```python
from build123d import *

# Parameters (mm, degrees)
BOSS_EXTRUDE1_DEPTH = 8


with BuildPart() as part:
    # Sketch1 → Boss-Extrude1 (new body)
    with BuildSketch(Plane.XY):
        with BuildLine():
            Line((1, 0), (19, 0))
            ThreePointArc((19, 0), (19.707106781, 0.292893219), (20, 1))
            Line((20, 1), (20, 56.5))
            ThreePointArc((20, 56.5), (19.707106781, 57.207106781), (19, 57.5))
            Line((19, 57.5), (1, 57.5))
            ThreePointArc((1, 57.5), (0.292893219, 57.207106781), (0, 56.5))
            Line((0, 56.5), (0, 50.5))
            ThreePointArc((0, 50.5), (0.292893219, 49.792893219), (1, 49.5))
            Line((1, 49.5), (10, 49.5))
            Line((10, 49.5), (10, 41.5))
            Line((10, 41.5), (1, 41.5))
            ThreePointArc((1, 41.5), (0.292893219, 41.207106781), (0, 40.5))
            Line((0, 40.5), (0, 19))
            ThreePointArc((0, 19), (0.292893219, 18.292893219), (1, 18))
            Line((1, 18), (10, 18))
            Line((10, 18), (10, 10))
            Line((10, 10), (1, 10))
            ThreePointArc((1, 10), (0.292893219, 9.707106781), (0, 9))
            Line((0, 9), (0, 1))
            ThreePointArc((0, 1), (0.292893219, 0.292893219), (1, 0))
        make_face()
    extrude(amount=BOSS_EXTRUDE1_DEPTH)


solid = part.part
```
Input: part model. Units: mm. Frame: model coordinates. A direction names the side the tool comes from. Coordinates: 2 decimals unless noted, no trailing zeros. Write each loop counter-clockwise with the first axis right and the second up, starting at its lowest first coordinate (ties: lowest second). Pieces come first, ordered by that corner, then holes. Notation, with made-up numbers: (3.5, 66) -> (22.5, 66) arc R15 cw to (22.5, 85) -> close; hole circle Ø8 at (64, 75.25). An arc over 180 degrees is marked (long way). Answer as a JSON object with one key per item and string values.
1. First-contact query: P1, Ø4, axis at y = 44, z = 6, coming from the -X side. Flat tip, straight axial feed; report the tip coordinate or a pass-through.
Result set:
{"P1": "stops at x = 10"}
2. Access query for faces 1 (the face through (0.301, 41.215, 3.944)), 2 (the face through (0, 30, 4)). Directions: +Z, -Z, +X, -X, +Y, -Y. A direction counts if a zero-diameter tool reaches every point of the face in a straight line with its end or side. Return the directions, or none.
Result set:
{"face 1": "+Z, -Z, -X", "face 2": "+Z, -Z, -X, +Y, -Y"}
3. Section A-A on x = 2.5. Return the cut outline in (y, z).
Result set:
{"outline": "(0, 0) -> (10, 0) -> (10, 8) -> (0, 8) -> close; (18, 0) -> (41.5, 0) -> (41.5, 8) -> (18, 8) -> close; (49.5, 0) -> (57.5, 0) -> (57.5, 8) -> (49.5, 8) -> close"}
4. Section C-C on y = 13.5. Return the cut outline in (x, z).
Result set:
{"outline": "(10, 0) -> (20, 0) -> (20, 8) -> (10, 8) -> close"}
5. Material intervals for line 1 (Y direction, x = 6.75, z = 2.5); line 2 (X direction, y = 45, z = 3.75); line 3 (X direction, y = 18.5, z = 6.5), sorted ascending. Write a range as from..to.
Result set:
{"line 1": "y = 0..10, 18..41.5, 49.5..57.5", "line 2": "x = 10..20", "line 3": "x = 0.13..20"}
6. Section B-B on z = 6. Return the cut outline in (x, y).
Result set:
{"outline": "(0, 1) arc R1 ccw to (1, 0) -> (19, 0) arc R1 ccw to (20, 1) -> (20, 56.5) arc R1 ccw to (19, 57.5) -> (1, 57.5) arc R1 ccw to (0, 56.5) -> (0, 50.5) arc R1 ccw to (1, 49.5) -> (10, 49.5) -> (10, 41.5) -> (1, 41.5) arc R1 ccw to (0, 40.5) -> (0, 19) arc R1 ccw to (1, 18) -> (10, 18) -> (10, 10) -> (1, 10) arc R1 ccw to (0, 9) -> close"}
